```python
from build123d import *

# Parameters (mm, degrees)
SKETCH1_W           = 80
SKETCH1_H           = 20
BOSS_EXTRUDE1_DEPTH = 5
FILLET1_R           = 5
SHELL1_T            = -2
SKETCH2_W           = 5
SKETCH2_H           = 5
BOSS_EXTRUDE2_DEPTH = 6
SKETCH3_R           = 1.425
CUT_EXTRUDE1_DEPTH  = 4


with BuildPart() as part:
    # Sketch1 → Boss-Extrude1 (new body)
    with BuildSketch(Plane.XY):
        Rectangle(SKETCH1_W, SKETCH1_H)
    extrude(amount=BOSS_EXTRUDE1_DEPTH)

    # Fillet1
    fillet1_edges = [part.edges().sort_by_distance(p)[0] for p in [
        (40, -10, 2.5),
        (-40, -10, 2.5),
        (-40, 10, 2.5),
        (40, 10, 2.5),
    ]]
    fillet(fillet1_edges, radius=FILLET1_R)

    # Shell1
    shell1_openings = [part.faces().sort_by_distance(p)[0] for p in [
        (0, 0, 0),
    ]]
    offset(amount=SHELL1_T, openings=shell1_openings, kind=Kind.INTERSECTION)

    # Sketch2 → Boss-Extrude2 (add)
    with BuildSketch(Plane(origin=(0, 10, 0), x_dir=(1, 0, 0), z_dir=(0, 1, 0))):
        with Locations((-3.653953893, -2.5)):
            Rectangle(SKETCH2_W, SKETCH2_H)
    extrude(amount=BOSS_EXTRUDE2_DEPTH)

    # Sketch3 → Cut-Extrude1 (cut)
    with BuildSketch(Plane(origin=(0, 16, 0), x_dir=(1, 0, 0), z_dir=(0, 1, 0))):
        with Locations((-3.653953893, -2.5)):
            Circle(SKETCH3_R)
    extrude(amount=-CUT_EXTRUDE1_DEPTH, mode=Mode.SUBTRACT)


solid = part.part
```
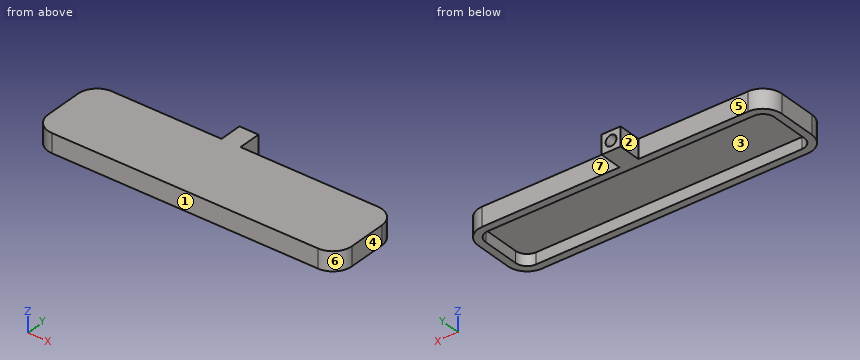
Can you work these out from the model? Positions are in its coordinate system, mm. Face numbers are marked on the shaded views. A direction names the side the tool comes from. Give positions to 0.01 mm unless a question says otherwise; leave off trailing zeros. Order: outer loops, then holes, each group sorted by start corner. A loop starts at its lowest first (then second) coordinate and runs counter-clockwise, first axis right, second up. Notation, with made-up numbers: (31, -26) - (57, -26) arc R27 ccw to (57, -4) - close; hole circle Ø6 at (11, -13.75). An arc over 180 degrees is marked (long way). Use a Markdown table: item, result. Add a question column.
Q1. If we section it at C-C on y = 11.25: Write out the boundary of the cut face in (x, z).
Q2. If we section it at A-A on z = 1.75: Write out the boundary of the cut face in (x, y).
Q3. If we mould it in two halves opening along X, with no side actions, what happens to the marked faces 1, 2, 3 and 4? For each: released by +X, released by -X, zero draft, split by the parting line, or undercut.
Q4. Please list where these lines run through material, in increasing order: line 1 along X through (y, z) = (3, 2.65); line 2 along X through (y, z) = (14.85, 2.5); line 3 along Y through (x, z) = (21.5, 1.9).
Q5. On a 3-axis mill with a long thin cutter (end or side, diameter ignored), from which of +Z, -Z, +X, -X, +Y, -Y can I reach the whole of each face in a straight line? I mean the marked faces 5, 6 and 7. Say none if no direction works.
Q6. If we section it at B-B on x = -22.5: Write out the boundary of the cut face in (y, z).
Q7. I'm going to push flat-ended pins straight in: pin 1 (1 mm diameter, centred on x = 11.5, z = 2, fed in from +Y); pin 2 (1.4 mm diameter, centred on x = -4, z = 2.5, fed in from +Y); pin 3 (13 mm diameter, centred on x = -17.5, y = 3.5, fed in from -Z); pin 4 (1 mm diameter, centred on x = -22.5, y = -6.5, fed in from -Z). Where does each tip first touch, or does it pass through?
Q8. If we section it at D-D on y = 6.5: Write out the boundary of the cut face in (x, z).
Answers follow:
| question | item | result |
|---|---|---|
| 1 | outline | (-6.15, 0) - (-1.15, 0) - (-1.15, 5) - (-6.15, 5) - close |
| 2 | outline | (-40, -5) arc R5 ccw to (-35, -10) - (35, -10) arc R5 ccw to (40, -5) - (40, 5) arc R5 ccw to (35, 10) - (-1.15, 10) - (-1.15, 16) - (-2.44, 16) - (-2.44, 12) - (-4.87, 12) - (-4.87, 16) - (-6.15, 16) - (-6.15, 10) - (-35, 10) arc R5 ccw to (-40, 5) - close; hole (-38, -5) arc R3 ccw to (-35, -8) - (35, -8) arc R3 ccw to (38, -5) - (38, 5) arc R3 ccw to (35, 8) - (-35, 8) arc R3 ccw to (-38, 5) - close |
| 3 | face 1 | zero draft |
| 3 | face 2 | released by -X |
| 3 | face 3 | undercut |
| 3 | face 4 | released by +X |
| 4 | line 1 | x = -40 to -38, 38 to 40 |
| 4 | line 2 | x = -6.15 to -5.08, -2.23 to -1.15 |
| 4 | line 3 | y = -10 to -8, 8 to 10 |
| 5 | face 5 | +Z, -Z, -X, +Y |
| 5 | face 6 | +Z, -Z, +X, -Y |
| 5 | face 7 | +Z, -Z, +X, +Y |
| 6 | outline | (-10, 0) - (-8, 0) - (-8, 3) - (8, 3) - (8, 0) - (10, 0) - (10, 5) - (-10, 5) - close |
| 7 | pin 1 | stops at y = 10 |
| 7 | pin 2 | stops at y = 12 |
| 7 | pin 3 | stops at z = 0 |
| 7 | pin 4 | stops at z = 3 |
| 8 | outline | (-39.77, 0) - (-37.6, 0) - (-37.6, 3) - (37.6, 3) - (37.6, 0) - (39.77, 0) - (39.77, 5) - (-39.77, 5) - close |
